Can you work these out from the model? Positions are in its coordinate system, mm. Face numbers are marked on the shaded views. A direction names the side the tool comes from. Give positions to 0.01 mm unless a question says otherwise; leave off trailing zeros. Order: outer loops, then holes, each group sorted by start corner. A loop starts at its lowest first (then second) coordinate and runs counter-clockwise, first axis right, second up. Notation, with made-up numbers: (20, -27.75) -> (49, -27.75) arc R35 cw to (49, 5.25) -> close; hole circle Ø10 at (4, -36.5). An arc over 180 degrees is marked (long way). Answer as a JSON object with one key per item and string values.
Autodesk Fusion 360 part; units mm, degrees
sketch "Sketch1" plane through (0, 0, 0) normal (0, 0, 1) x (1, 0, 0)
  line L0 (112.5, -100) -> (-112.5, -100)
  line L1 (-112.5, -100) -> (-112.5, 100)
  line L2 (-112.5, 100) -> (112.5, 100)
  line L3 (112.5, 100) -> (112.5, -100)
  line L4 (112.5, -100) -> (-112.5, 100) construction
  line L5 (-112.5, -100) -> (112.5, 100) construction
  line L6 (0, 100) -> (0, -100) construction
  line L7 (-112.5, 0) -> (112.5, 0) construction
  dimension "d1" = 225
  dimension "d2" = 200
extrude "Extrude1" add sketch "Sketch1" along normal blind 150
sketch "Sketch2" plane through (0, 100, 0) normal (0, 1, 0) x (-1, 0, 0)
  line L0 (-112.5, 0) -> (112.5, 0)
  line L1 (112.5, 0) -> (112.5, 150)
  line L2 (112.5, 150) -> (-112.5, 150)
  line L3 (-112.5, 150) -> (-112.5, 0)
  line L4 (112.5, 150) -> (37.5, 150)
  line L5 (37.5, 150) -> (37.5, 40)
  line L6 (37.5, 40) -> (112.5, 40)
  line L7 (112.5, 40) -> (112.5, 150)
  dimension "d5" = 75
sketch "Sketch3" plane through (0, 100, 0) normal (0, 1, 0) x (-1, 0, 0)
extrude "Extrude2" cut sketch "Sketch2" against normal blind 540 contours L1 L2 L4 L5 L6 L7
sketch "Sketch4" plane through (0, 100, 0) normal (0, 1, 0) x (-1, 0, 0)
  line L0 (112.5, 40) -> (37.5, 40)
  line L1 (37.5, 40) -> (37.5, 150)
  line L2 (37.5, 150) -> (-112.5, 150)
  line L3 (-112.5, 150) -> (-112.5, 0)
  line L4 (-112.5, 0) -> (112.5, 0)
  line L5 (112.5, 0) -> (112.5, 40)
sketch "Sketch5" plane through (0, 0, 150) normal (0, 0, 1) x (-1, 0, 0)
  line L0 (37.5, -100) -> (37.5, 100)
  line L1 (37.5, 100) -> (-112.5, 100)
  line L2 (-112.5, 100) -> (-112.5, -100)
  line L3 (-112.5, -100) -> (37.5, -100)
sketch "Sketch6" plane through (0, 100, 0) normal (0, 1, 0) x (-1, 0, 0)
  line L0 (-112.5, 0) -> (-112.5, 70)
  line L1 (-112.5, 70) -> (-90, 70)
  line L2 (-90, 70) -> (-90, 100)
  line L3 (-90, 100) -> (-30, 100)
  line L4 (-30, 100) -> (-30, 0)
  line L5 (-30, 0) -> (-112.5, 0)
  line L6 (37.5, 150) -> (-112.5, 150)
  point P0 (37.5, 150)
  point P1 (37.5, 40)
  point P2 (-112.5, 0)
  dimension "d8" = 50
  dimension "d9" = 80
  dimension "d10" = 110
  dimension "d11" = 150
extrude "Extrude3" cut sketch "Sketch6" against normal blind 375
sketch "Sketch7" plane through (0, 0, 150) normal (0, 0, 1) x (-1, 0, 0)
  line L0 (-37.5, 100) -> (-37.5, -100) construction
  line L1 (-112.7809, 55) -> (35.5051, 55) construction
  line L2 (-110, -55) -> (40, -55) construction
  point P0 (-112.5, 100)
  point P1 (37.5, -100)
  dimension "d14" = 75
  dimension "d15" = 45
  dimension "d16" = 45
sketch "Sketch8" plane through (0, 0, 150) normal (0, 0, 1) x (-1, 0, 0)
  line L0 (-37.5, 100) -> (-37.5, -100)
  point P0 (-112.5, -100)
  dimension "d17" = 75
sketch "Sketch9" plane through (0, 100, 0) normal (0, 1, 0) x (-1, 0, 0)
  point P0 (-112.7809, 150)
  point P1 (37.5, 150)
sketch "Sketch10" plane through (0, 0, 150) normal (0, 0, 1) x (-1, 0, 0)
  line L0 (-111.7438, 55) -> (36.0063, 55)
  line L1 (112.5, 0) -> (-112.3459, 0) construction
  line L2 (40, -55) -> (-112.822, -55) construction
  point P0 (-112.5, 100)
  point P1 (-37.5, 100)
  point P2 (-112.5, 100)
  point P3 (40, -55)
  point P4 (37.5, -100)
  dimension "d19" = 75
  dimension "d20" = 45
  dimension "d21" = 45
sketch "Sketch11" plane through (0, 0, 150) normal (0, 0, 1) x (-1, 0, 0)
hole "Hole1" at (36.2725, -54.6667, 150) direction (0, 0, -1) diameter 30 depth 50 tip angle 180 counterbore diameter 50 counterbore depth 20
hole "Hole2" at (36.4807, 55.0076, 150) direction (0, 0, -1) diameter 30 depth 50 tip angle 180 counterbore diameter 50 counterbore depth 20
sketch "Sketch12" plane through (0, 0, 40) normal (0, 0, 1) x (-1, 0, 0)
  line L0 (112.5, 100) -> (37.5, 100)
  line L1 (37.5, 100) -> (37.5, -100)
  line L2 (37.5, -100) -> (112.5, -100)
  line L3 (112.5, -100) -> (112.5, 100)
sketch "Sketch13" plane through (0, 0, 40) normal (0, 0, 1) x (-1, 0, 0)
sketch "Sketch14" plane through (0, 0, 40) normal (0, 0, 1) x (-1, 0, 0)
sketch "Sketch15" plane through (0, 0, 40) normal (0, 0, 1) x (-1, 0, 0)
sketch "Sketch16" plane through (0, 0, 40) normal (0, 0, 1) x (-1, 0, 0)
  line L0 (112.5, -100) -> (112.5, 100)
  line L1 (112.5, 100) -> (162.5, 100)
  line L2 (162.5, 100) -> (162.5, -100)
  line L3 (162.5, -100) -> (112.5, -100)
  dimension "d40" = 50
  dimension "d41" = 200
  dimension "d42" = 50
extrude "Extrude4" add sketch "Sketch16" against normal blind 40
sketch "Sketch17" plane through (0, 0, 40) normal (0, 0, 1) x (-1, 0, 0)
  line L0 (112.5, 100) -> (37.5, 100)
  line L1 (37.5, 100) -> (37.5, -100)
  line L2 (37.5, -100) -> (112.5, -100)
  line L3 (112.5, -100) -> (162.5, -100)
  line L4 (162.5, -100) -> (162.5, 100)
  line L5 (162.5, 100) -> (112.5, 100)
sketch "Sketch18" plane through (0, 0, 40) normal (0, 0, 1) x (-1, 0, 0)
  line L0 (162.3989, 55) -> (162.5, 55)
  line L1 (162.5, -55) -> (162.485, -55)
  line L2 (162.5, -55) -> (162.5, -100)
  line L3 (162.5, -100) -> (112.5, -100)
  line L4 (162.5, -100) -> (112.5, -100)
  line L5 (112.5, -100) -> (162.5, -55)
  line L6 (112.5, 0) -> (-112.3459, 0)
  line L7 (162.5, 100) -> (112.5, 100)
  line L8 (112.5, 100) -> (162.5, 55)
  line L9 (162.5, 55) -> (162.5, 100)
  point P0 (162.5, -100)
  point P1 (162.5, 100)
  dimension "d45" = 45
  dimension "d46" = 45
  dimension "d47" = 50
  dimension "d48" = 50
extrude "Extrude5" cut sketch "Sketch18" against normal blind 40
sketch "Sketch19" plane through (0, 0, 40) normal (0, 0, 1) x (-1, 0, 0)
  line L0 (162.5, -55) -> (232.5, -55)
  line L1 (162.5, 55) -> (232.5, 55)
  line L2 (162.5, -55) -> (162.5, 55)
  circle A0 centre (232.5, 0) radius 25
  arc A1 (232.5, -55) -> (232.5, 55) centre (232.5, 0) ccw
  line L3 (162.5, -100) -> (162.5, 100)
  point P0 (37.5, 100)
  point P1 (37.5, -100)
  dimension "d51" = 70
  dimension "d52" = 70
  dimension "d53" = 45
  dimension "d54" = 45
  dimension "d55" = 50
extrude "Extrude6" add sketch "Sketch19" against normal blind 40
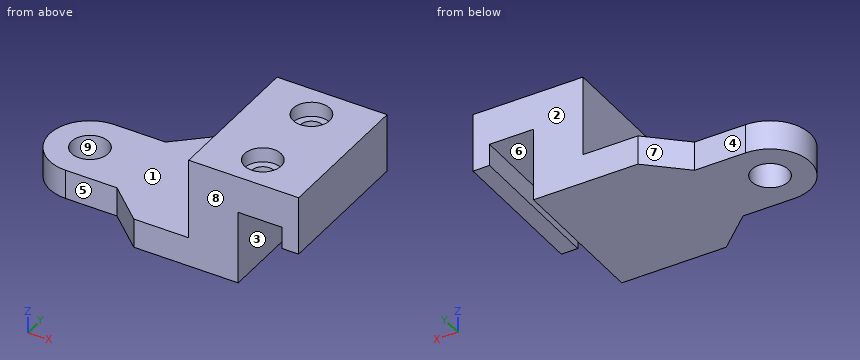
1. If we section it at C-C on z = 23: Please give me the cut outline in (x, y).
Worked answers:
{"outline": "(-232.5, -55) -> (-162.5, -55) -> (-112.5, -100) -> (30, -100) -> (30, 100) -> (-112.5, 100) -> (-162.5, 55) -> (-232.5, 55) arc R55 ccw to start; hole circle Ø50 at (-232.5, 0)"}
2. If we section it at A-A on z = 88.5: Please give me the cut outline in (x, y).
Worked answers:
{"outline": "(-37.5, -100) -> (30, -100) -> (30, 100) -> (-37.5, 100) -> close; (90, -100) -> (112.5, -100) -> (112.5, 100) -> (90, 100) -> close"}
3. Will these pins go through, and if not, where does the flat tip stop? pin 1 Ø6 at (y, z) = (-33, 54.5) entering from +X; pin 2 Ø24 at (x, y) = (36.48, 55.01) entering from +Z; pin 3 Ø11 at (x, y) = (104, 7.5) entering from -Z; pin 4 Ø1.5 at (x, z) = (-38.5, 106) entering from -Y.
Worked answers:
{"pin 1": "x = 30", "pin 2": "z = 100", "pin 3": "z = 70", "pin 4": "through"}
4. If we mould it in two halves opening along Y, with no side actions, what happens to the marked faces 6, 7, 8 and 9? For each: +Y half, -Y half, draft (parallel to the pull), parting line (faces both ways), or undercut.
Worked answers:
{"face 6": "draft", "face 7": "+Y half", "face 8": "-Y half", "face 9": "undercut"}
5. For the marked faces 1, 2, 3, 4 and 5, which set-ups out of +Z, -Z, +X, -X, +Y, -Y let a thin tool reach every point of the face, with its end or its side?
Worked answers:
{"face 1": "+Z, -X, +Y, -Y", "face 2": "+Z, -Z, +X, -X, +Y", "face 3": "-Z, +Y, -Y", "face 4": "+Z, -Z, -X, +Y", "face 5": "+Z, -Z, -X, -Y"}
6. If we section it at D-D on y = -20.5: Please give me the cut outline in (x, z), then the cut area to 3 significant figures.
Worked answers:
{"outline": "(-283.54, 0) -> (-246.81, 0) -> (-246.81, 40) -> (-283.54, 40) -> close; (-218.19, 0) -> (30, 0) -> (30, 100) -> (90, 100) -> (90, 70) -> (112.5, 70) -> (112.5, 150) -> (-37.5, 150) -> (-37.5, 40) -> (-218.19, 40) -> close", "area": "23,600 mm²"}
7. Please list where these lines run through material, in increasing order: L1, parallel to X at y = -19, z = 90; L2, parallel to Y at x = 33.5, z = 136.5; L3, parallel to Z at x = -72, y = 88.
Worked answers:
{"L1": "-37.5 to 30, 90 to 112.5", "L2": "-100 to -79.51, -29.82 to 30.19, 79.83 to 100", "L3": "0 to 40"}
8. If we section it at B-B on y = 0: Please give me the cut outline in (x, z).
Worked answers:
{"outline": "(-287.5, 0) -> (-257.5, 0) -> (-257.5, 40) -> (-287.5, 40) -> close; (-207.5, 0) -> (30, 0) -> (30, 100) -> (90, 100) -> (90, 70) -> (112.5, 70) -> (112.5, 150) -> (-37.5, 150) -> (-37.5, 40) -> (-207.5, 40) -> close"}
